```python
from build123d import *

# Parameters (mm, degrees)
SKETCH1_W           = 26.5
SKETCH1_H           = 22.4
BOSS_EXTRUDE1_DEPTH = 2
BOSS_EXTRUDE2_DEPTH = 22.4


with BuildPart() as part:
    # Sketch1 → Boss-Extrude1 (new body)
    with BuildSketch(Plane.XY):
        Rectangle(SKETCH1_W, SKETCH1_H)
    extrude(amount=BOSS_EXTRUDE1_DEPTH)

    # Sketch2 → Boss-Extrude2 (add)
    with BuildSketch(Plane(origin=(0, 11.2, 0), x_dir=(1, 0, 0), z_dir=(0, 1, 0))):
        with BuildLine():
            Line((13.25, -2), (-12.347034397, -8.858704695))
            ThreePointArc((-12.347034397, -8.858704695), (-13.023288826, -5.458944094), (-13.25, -2))
            Line((-13.25, -2), (13.25, -2))
        make_face()
    extrude(amount=-BOSS_EXTRUDE2_DEPTH)


solid = part.part
```
Verification items for the finished model (mm, model axes). Coordinates: 2 decimals unless noted, no trailing zeros. Loops run counter-clockwise (first coordinate to the right, second up) from the corner with the lowest first, then second, coordinate; pieces in that order, holes last. Notation, with made-up numbers: (65.25, -23) -> (112.25, -23) arc R13 ccw to (112.25, -3) -> close; hole circle Ø7 at (-32, 72.25). An arc over 180 degrees is marked (long way). Put each result on its own line as item: value.
1. Section check A-A, the plane y = -8. Record the boundary of the cut face in (x, z), then the cut area to 3 significant figures.
Result set:
outline: (-13.25, 0) -> (13.25, 0) -> (13.25, 2) -> (-12.35, 8.86) arc R26.5 ccw to (-13.25, 2) -> close
area: 145 mm^2
2. Section check B-B, the plane x = -10. Record the boundary of the cut face in (y, z), then the cut area to 3 significant figures.
Result set:
outline: (-11.2, 0) -> (11.2, 0) -> (11.2, 8.23) -> (-11.2, 8.23) -> close
area: 184 mm^2
3. Gauge pin test, flat ends, axial feed: P1, Ø4, axis at x = 6, y = -7, coming from the +Z side; P2, Ø3, axis at x = -7.5, y = 4.5, coming from the +Z side. Record the tip position at first contact, or that the pin passes through.
Result set:
P1: stops at z = 4.48
P2: stops at z = 7.96
4. Section check C-C, the plane z = 3. Record the boundary of the cut face in (x, y).
Result set:
outline: (-13.23, -11.2) -> (9.52, -11.2) -> (9.52, 11.2) -> (-13.23, 11.2) -> close
5. Thickness scan on line 1 (Z direction, x = -4, y = 1.25); line 2 (Z direction, x = -6.75, y = -9.5). Record the ranges inside material, lowest first.
Result set:
line 1: z = 0 to 6.62
line 2: z = 0 to 7.36
